Can you work these out from the drawing? Everything is in mm from the part's minimum corner. A direction names the side the tool comes from. Coordinates: 2 decimals unless noted, no trailing zeros. Loops run counter-clockwise (first coordinate to the right, second up) from the corner with the lowest first, then second, coordinate; pieces in that order, holes last. Notation, with made-up numbers: (-22.5, 87.25) - (-9.5, 87.25) arc R16 ccw to (-9.5, 93.25) - close; hole circle Ø4 at (3.25, 56). An arc over 180 degrees is marked (long way). One line per question, with ' | ' between items. Start each with the question number.
1. Which directions (+Z, -Z, +X, -X, +Y, -Y) give clear straight access to the entire face, cutting with the end or side of a thin tool? Please do the marked faces 1, 2 and 3.
2. Please list where these lines run through material, in increasing order: L1, parallel to Y at x = 3.5, z = 101; L2, parallel to Z at x = 10, y = 39; L3, parallel to X at y = 24, z = 67.5. Write a range as [from, to].
3. I want a section at D-D, the plane x = 41.5. Write out the boundary of the cut face in (y, z).
4. I want a section at B-B, the plane z = 49.5. Write out the boundary of the cut face in (x, y), then the cut area to 3 significant figures.
5. I'm going to push flat-ended pins straight in: P1, Ø1, axis at y = 36, z = 46, coming from the +X side; P2, Ø1.6, axis at x = 29.5, y = 24.5, coming from the +Z side; P3, Ø0.6, axis at y = 24.5, z = 70, coming from the -X side; P4, Ø10, axis at x = 13, y = 40.5, coming from the -Z side. Where does each tip first touch, or does it pass through?
6. I want a section at A-A, the plane x = 30. Write out the boundary of the cut face in (y, z).
7. I want a section at C-C, the plane y = 30. Write out the boundary of the cut face in (x, z).
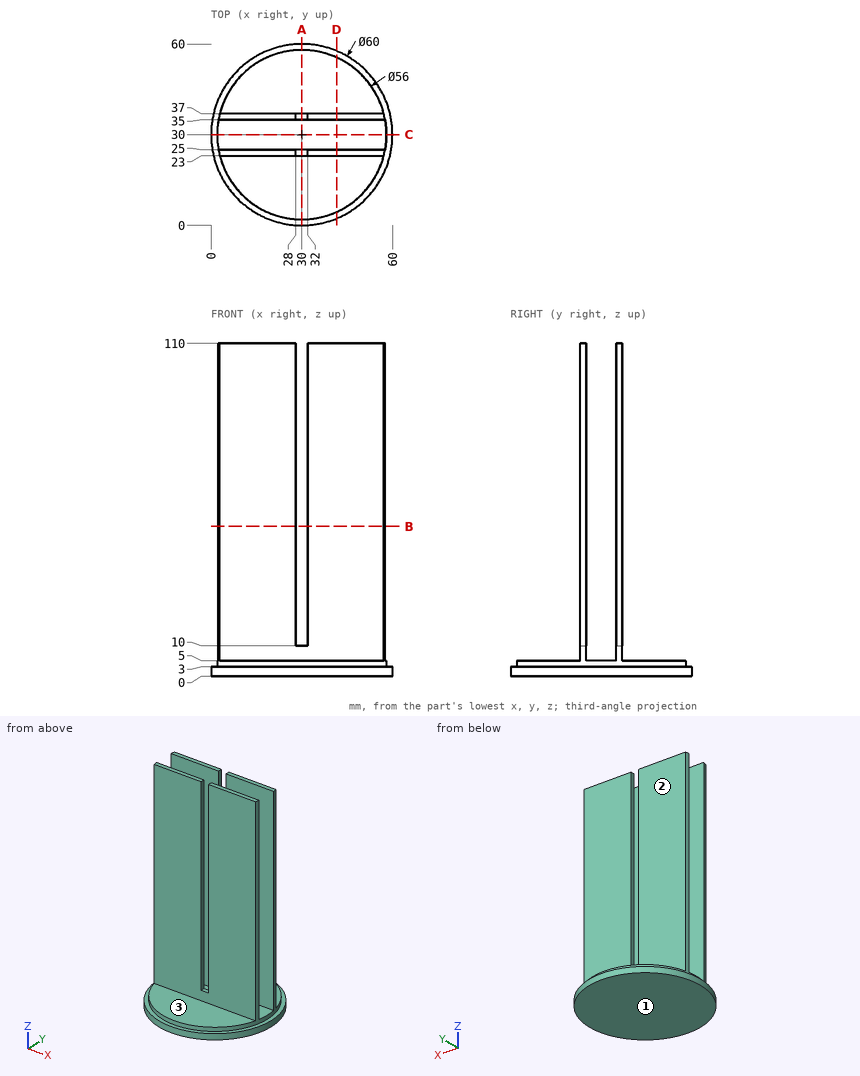
Results are:
1) face 1: -Z, +X, -X, +Y, -Y | face 2: +Z, +X, -X, +Y | face 3: +Z, +X, -X, -Y
2) L1: y = [23, 25], [35, 37] | L2: z = [0, 5] | L3: x = [2.65, 28], [32, 57.35]
3) outline: (2.29, 0) - (57.71, 0) - (57.71, 3) - (55.53, 3) - (55.53, 5) - (37, 5) - (37, 110) - (35, 110) - (35, 5) - (25, 5) - (25, 110) - (23, 110) - (23, 5) - (4.47, 5) - (4.47, 3) - (2.29, 3) - close
4) outline: (2.45, 25) arc R28 ccw to (2.89, 23) - (28, 23) - (28, 25) - close; (2.45, 35) - (28, 35) - (28, 37) - (2.89, 37) arc R28 ccw to start; (32, 23) - (57.11, 23) arc R28 ccw to (57.55, 25) - (32, 25) - close; (32, 35) - (57.55, 35) arc R28 ccw to (57.11, 37) - (32, 37) - close | area: 203 mm2
5) P1: stops at x = 57.45 | P2: stops at z = 10 | P3: stops at x = 2.49 | P4: stops at z = 0
6) outline: (0, 0) - (60, 0) - (60, 3) - (58, 3) - (58, 5) - (37, 5) - (37, 10) - (35, 10) - (35, 5) - (25, 5) - (25, 10) - (23, 10) - (23, 5) - (2, 5) - (2, 3) - (0, 3) - close
7) outline: (0, 0) - (60, 0) - (60, 3) - (58, 3) - (58, 5) - (2, 5) - (2, 3) - (0, 3) - close
